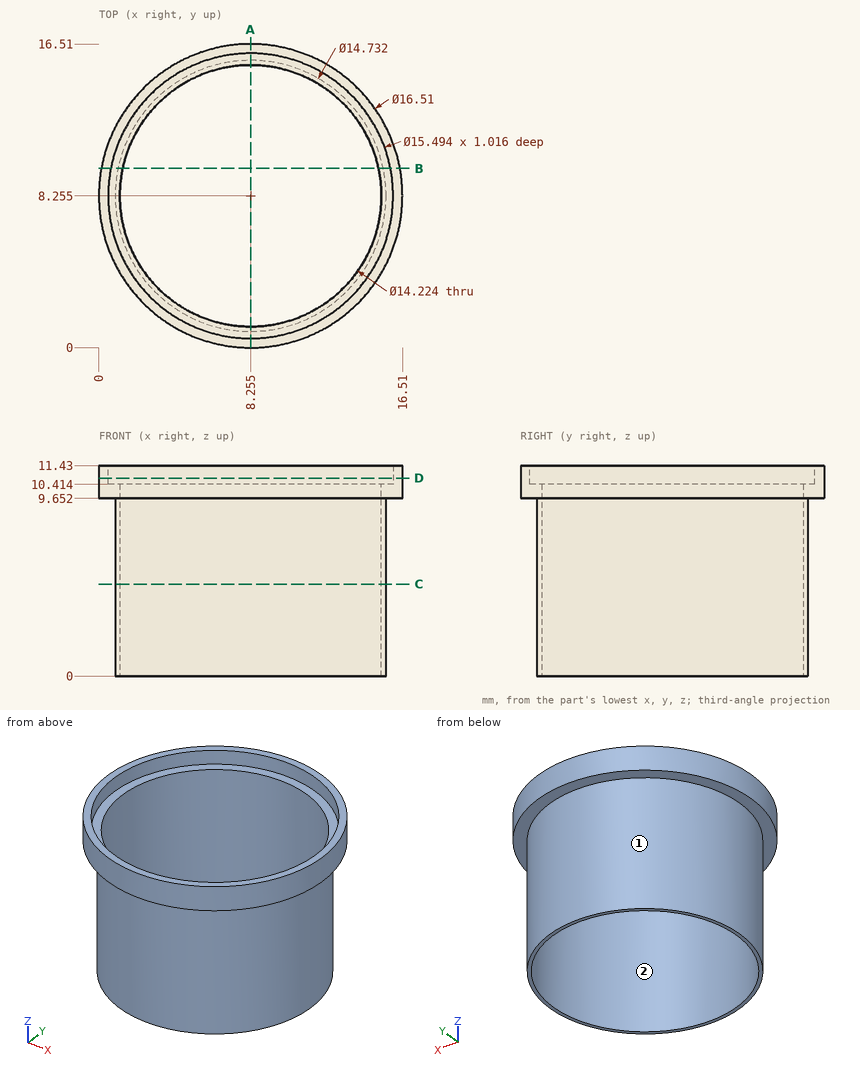
Geometry check sheet. Reference: drawing and pictorial views, mm from the part's lowest x, y, z. Round coordinates to 2 decimals unless told otherwise and drop trailing zeros. Order: outer loops, then holes, each group sorted by start corner. A loop starts at its lowest first (then second) coordinate and runs counter-clockwise, first axis right, second up. Notation, with made-up numbers: (45.5, -7) - (61.5, -7) arc R24 ccw to (61.5, 27) - close; hole circle Ø5 at (-4.75, 61). An arc over 180 degrees is marked (long way). One line per question, with ' | ' between items. Start each with the question number.
(1) Sectioned sample at B-B on y = 9.75. Record the cut outline in (x, z).
(2) Release check for a two-part mould opening along X. For the marked faces 1 and 2 record: released by +X, released by -X, zero draft, split by the parting line, or undercut.
(3) Sectioned sample at D-D on z = 10.75. Record the cut outline in (x, y) (3 decimals).
(4) Depth check by flat-ended pin: pin 1 Ø4 at (x, y) = (3, 9.5) entering from +Z; pin 2 Ø6 at (x, z) = (2, 6.5) entering from +Y; pin 3 Ø1.5 at (y, z) = (13, 4.5) entering from +X; pin 4 Ø5 at (y, z) = (8.5, 8) entering from +X. Enter the tip coordinate at first touch or a pass-through.
(5) Thickness scan on L1, parallel to Y at x = 8.5, z = 8.5; L2, parallel to Z at x = 2.5, y = 14; L3, parallel to X at y = 13.5, z = 2. Record the ranges inside material, lowest first. Write a range as [from, to].
(6) Sectioned sample at C-C on z = 5. Record the cut outline in (x, y) (3 decimals).
(7) Sectioned sample at A-A on x = 8.25. Record the cut outline in (y, z), and give its area (3 significant figures).
Conclusion:
1) outline: (0.14, 9.65) - (1.04, 9.65) - (1.04, 0) - (1.3, 0) - (1.3, 10.41) - (0.65, 10.41) - (0.65, 11.43) - (0.14, 11.43) - close; (15.21, 0) - (15.47, 0) - (15.47, 9.65) - (16.37, 9.65) - (16.37, 11.43) - (15.86, 11.43) - (15.86, 10.41) - (15.21, 10.41) - close
2) face 1: split by the parting line | face 2: undercut
3) outline: circle Ø16.51 at (8.255, 8.255); hole circle Ø15.494 at (8.255, 8.255)
4) pin 1: stops at z = 10.41 | pin 2: stops at y = 14.86 | pin 3: stops at x = 14.44 | pin 4: stops at x = 16.51
5) L1: y = [0.89, 1.15], [15.36, 15.62] | L2: z = [9.65, 11.43] | L3: x = [3.08, 3.45], [13.06, 13.43]
6) outline: circle Ø14.732 at (8.255, 8.255); hole circle Ø14.224 at (8.255, 8.255)
7) outline: (0, 9.65) - (0.89, 9.65) - (0.89, 0) - (1.14, 0) - (1.14, 10.41) - (0.51, 10.41) - (0.51, 11.43) - (0, 11.43) - close; (15.37, 0) - (15.62, 0) - (15.62, 9.65) - (16.51, 9.65) - (16.51, 11.43) - (16, 11.43) - (16, 10.41) - (15.37, 10.41) - close | area: 7.68 mm2
